The listing builds one solid part. Answer for the finished solid, in the listing's coordinates (mm). A direction names the side the tool comes from. Give positions to 0.01 mm unless a question says otherwise; leave off trailing zeros. Order: outer loops, then holes, each group sorted by start corner. A loop starts at its lowest first (then second) coordinate and runs counter-clockwise, first axis right, second up. Notation, with made-up numbers: (86.25, 19) - (101.25, 19) arc R10 cw to (101.25, 24) - close; hole circle Ø8 at (83.5, 51.25). An arc over 180 degrees is marked (long way). Use a Markdown table: item, result. Add a question column.
1) Find section A-A, the plane x = 0. Determine the outline of the cut face in (y, z), plus the area to 3 significant figures.
2) The mould has two halves that part along Z. Classify faces 1 (the face through (12, -13, -40)), 2 (the face through (0, 0, 220)), 3 (the face through (-22.48, 0.99, 85.79)): released by +Z, released by -Z, zero draft, split by the parting line, or undercut.
3) Find section D-D, the plane x = -237. Determine the outline of the cut face in (y, z).
4) Flat-ended cylindrical pins translate along their axes: pin 1 (5 mm diameter, centred on x = 26.5, y = 6.5, fed in from +Z); pin 2 (2 mm diameter, centred on x = -35, y = -1, fed in from -Z); pin 3 (1 mm diameter, centred on x = 525.5, z = -36.5, fed in from +Y). Find the tip coordinate at first contact, or state that the pin passes through.
5) Find section B-B, the plane z = 0. Determine the outline of the cut face in (x, y).
6) For faces 4 (the face through (73, -12.5, 76)), 5 (the face through (-13.887, -10.648, -74.51)), 6 (the face through (11.62, 21.5, 33.73)), determine the directions among +Z, -Z, +X, -X, +Y, -Y from which every point of the face is accessible in a straight line to the end or side of a thin tool.
7) Find section C-C, the plane z = -63. Determine the outline of the cut face in (x, y), plus the area to 3 significant figures.
8) Straight lines are drawn through the part: line 1 (Z direction, x = 361, y = 0); line 2 (X direction, y = -2.5, z = 60); line 3 (X direction, y = 12, z = 78). For each, find the intervals that lie inside material, in ascending order.
from build123d import *

# Parameters (mm, degrees)
F0_R          = 40
F1_DEPTH      = 830
F1_DEPTH_BACK = 830
F2_R          = 22.5
F3_DEPTH      = 140
F3_DEPTH_BACK = 40
F4_R          = 17.5
F5_DEPTH      = 80
F5_DEPTH_BACK = 250
F7_DEPTH      = 12.5
F8_R          = 35.000000149
F9_DEPTH      = 1660.0010001


# Not quite as in the source:
# - a pattern or mirror of a feature is missing from the dataset's text; its kind, count and spacing are read off the source's solid


with BuildPart() as f1:
    # F0 (on Right) → F1 (new body, two sides)
    with BuildSketch(Plane.YZ) as f1_sk:
        Circle(F0_R)
    extrude(amount=F1_DEPTH)
    extrude(f1_sk.sketch, amount=-F1_DEPTH_BACK)

    # F2 (on Top) → F3 (join, two sides)
    with BuildSketch(Plane.XY) as f3_sk:
        Circle(F2_R)
    extrude(amount=F3_DEPTH)
    extrude(f3_sk.sketch, amount=-F3_DEPTH_BACK)

    # F4 (on face) → F5 (join, two sides)
    with BuildSketch(Plane.XY.offset(140)) as f5_sk:
        Circle(F4_R)
    extrude(amount=F5_DEPTH)
    extrude(f5_sk.sketch, amount=-F5_DEPTH_BACK)

    # F6 (on Front) → F7 (join, symmetric)
    with BuildSketch(Plane.XZ):
        Polygon((0, 109.4836109607), (0, 140), (-200, 0), (-156.4051585152, 0), align=None)
    f7 = extrude(amount=F7_DEPTH, both=True)

    # F7_copies: F7 across plane
    add(f7.mirror(Plane(origin=(0, 0, 0), x_dir=(0, 0, 1), z_dir=(1, 0, 0))))

    # F8 (on face) → F9 (cut, through all)
    with BuildSketch(Plane(origin=(-830, 0, 0), x_dir=(0, -1, 0), z_dir=(-1, 0, 0))):
        Circle(F8_R)
    extrude(amount=-F9_DEPTH, mode=Mode.SUBTRACT)


solid = f1.part
The answers:
| question | item | result |
|---|---|---|
| 1 | outline | (-22.5, -40) - (-17.5, -40) - (-17.5, -110) - (17.5, -110) - (17.5, -40) - (22.5, -40) - (22.5, -33.07) arc R40 ccw to (22.5, 33.07) - (22.5, 140) - (17.5, 140) - (17.5, 220) - (-17.5, 220) - (-17.5, 140) - (-22.5, 140) - (-22.5, 33.07) arc R40 ccw to (-22.5, -33.07) - close; hole circle Ø70 at (0, 0) |
| 1 | area | 11,100 mm2 |
| 2 | face 1 | released by -Z |
| 2 | face 2 | released by +Z |
| 2 | face 3 | undercut |
| 3 | outline | circle Ø80 at (0, 0); hole circle Ø70 at (0, 0) |
| 4 | pin 1 | z = 123.2 |
| 4 | pin 2 | z = -40 |
| 4 | pin 3 | y = 17.44 |
| 5 | outline | (-830, -40) - (830, -40) - (830, -35) - (-830, -35) - close; (-830, 35) - (830, 35) - (830, 40) - (-830, 40) - close |
| 6 | face 4 | +Z, +X, -Y |
| 6 | face 5 | -Z |
| 6 | face 6 | none |
| 7 | outline | circle Ø35 at (0, 0) |
| 7 | area | 962 mm2 |
| 8 | line 1 | -40 to -35, 35 to 40 |
| 8 | line 2 | -114.29 to -70.69, -22.36 to 22.36, 70.69 to 114.29 |
| 8 | line 3 | -88.57 to -44.98, -19.03 to 19.03, 44.98 to 88.57 |
